CAD build for the part. Positions are in the model's coordinates, mm. A direction names the side the tool comes from. Coordinates: 2 decimals unless noted, no trailing zeros. Order: outer loops, then holes, each group sorted by start corner. A loop starts at its lowest first (then second) coordinate and runs counter-clockwise, first axis right, second up. Notation, with made-up numbers: M 5,66.25 L 55,66.25 A30 cw 55,91.25 Z; hole C 9,44.25 d7. An arc over 180 degrees is marked long. Write item = value, one per line.
from build123d import *

# Parameters (mm, degrees)
SKETCH_W        = 28
SKETCH_H        = 20
SKETCH_R        = 1.75
PAD_DEPTH       = 4
PAD001_DEPTH    = 6
SKETCH002_R     = 3.25
POCKET_DEPTH    = 10
POCKET001_DEPTH = 7
SKETCH004_R     = 8.25
POCKET002_DEPTH = 2


with BuildPart() as part:
    # Sketch → Pad (new body)
    with BuildSketch(Plane.XY):
        Rectangle(SKETCH_W, SKETCH_H)
        with Locations((-11, 0)):
            Circle(SKETCH_R, mode=Mode.SUBTRACT)
        with Locations((11, 0)):
            Circle(SKETCH_R, mode=Mode.SUBTRACT)
    extrude(amount=PAD_DEPTH)

    # Sketch001 (on Face8 of Pad) → Pad001 (join)
    with BuildSketch(Plane.XY.offset(4)):
        with BuildLine():
            ThreePointArc((14, 1.802776), (7.5, 0), (14, -1.802776))
            Line((14, -1.802776), (14, -10))
            Line((14, -10), (-14, -10))
            Line((-14, -10), (-14, -1.802776))
            ThreePointArc((-14, -1.802776), (-7.5, 0), (-14, 1.802776))
            Line((-14, 1.802776), (-14, 10))
            Line((-14, 10), (14, 10))
            Line((14, 10), (14, 1.802776))
        make_face()
    extrude(amount=PAD001_DEPTH)

    # Sketch002 (on Face15 of Pad001) → Pocket (cut)
    with BuildSketch(Plane.XY.offset(10)):
        with Locations((0, 2)):
            Circle(SKETCH002_R)
    extrude(amount=-POCKET_DEPTH, mode=Mode.SUBTRACT)

    # Sketch003 (on Face4 of Pocket) → Pocket001 (cut)
    with BuildSketch(Plane(origin=(0, 0, 0), x_dir=(1, 0, 0), z_dir=(0, 0, -1))):
        Polygon((4.25, -4.453739), (4.25, 0.453739), (0, 2.907477), (-4.25, 0.453739), (-4.25, -4.453739), (0, -6.907477), align=None)
    extrude(amount=-POCKET001_DEPTH, mode=Mode.SUBTRACT)

    # Sketch004 (on Face4 of Pocket001) → Pocket002 (cut)
    with BuildSketch(Plane(origin=(0, 0, 0), x_dir=(1, 0, 0), z_dir=(0, 0, -1))):
        with Locations((0, -2)):
            Circle(SKETCH004_R)
    extrude(amount=-POCKET002_DEPTH, mode=Mode.SUBTRACT)


solid = part.part
(1) Tool access for faces 4 (the face through (0, -2, 10)), 5 (the face through (2, 5, 7)), 6 (the face through (-9, -1, 4)): list every direction of +Z, -Z, +X, -X, +Y, -Y with a clear straight run to the whole face (end or side of a thin tool).
Evaluation:
face_4 = +Z, +X, -X, +Y, -Y
face_5 = -Z
face_6 = +Z
(2) Pull direction X, two halves, no side cores. Call faces 1 (the face through (-2, -2, 2)), 2 (the face through (0, -10, 5)), 3 (the face through (14, 0.1, 3.8)): +X half, -X half, draft (parallel to the pull), parting line (faces both ways), or undercut.
Evaluation:
face_1 = undercut
face_2 = draft
face_3 = +X half
(3) Wall check: line 1 (Y direction, x = 11, z = 3.25); line 2 (X direction, y = -0.75, z = 3.25); line 3 (X direction, y = 2, z = 0.7). Give the ranges that are in metal, low to high. Write a range as from..to.
Evaluation:
line_1 = -10..-1.75, 1.75..10
line_2 = -14..-12.58, -9.42..-3.74, 3.74..9.42, 12.58..14
line_3 = -14..-8.25, 8.25..14
(4) Slice it at A-A, the plane x = -11. Write the cut outline in (y, z).
Evaluation:
outline = M -10,0 L -1.75,0 L -1.75,4 L -3.5,4 L -3.5,10 L -10,10 Z; M 1.75,0 L 10,0 L 10,10 L 3.5,10 L 3.5,4 L 1.75,4 Z
(5) Slice it at C-C, the plane x = 0.75. Write the cut outline in (y, z).
Evaluation:
outline = M -10,0 L -6.22,0 L -6.22,2 L -2.47,2 L -2.47,7 L -1.16,7 L -1.16,10 L -10,10 Z; M 5.16,7 L 6.47,7 L 6.47,2 L 10,2 L 10,10 L 5.16,10 Z
(6) Slice it at B-B, the plane y = 0.75. Write the cut outline in (x, z).
Evaluation:
outline = M -14,0 L -12.58,0 L -12.58,4 L -14,4 Z; M -9.42,0 L -8.15,0 L -8.15,2 L -4.25,2 L -4.25,7 L -3,7 L -3,10 L -7.58,10 L -7.58,4 L -9.42,4 Z; M 3,7 L 4.25,7 L 4.25,2 L 8.15,2 L 8.15,0 L 9.42,0 L 9.42,4 L 7.58,4 L 7.58,10 L 3,10 Z; M 12.58,0 L 14,0 L 14,4 L 12.58,4 Z
(7) Pin check, flat tips, straight feed: pin 1 Ø4.5 at (x, y) = (0.5, 1.5) entering from -Z; pin 2 Ø6 at (x, y) = (2.5, -5) entering from -Z; pin 3 Ø2 at (x, y) = (-12, 1.5) entering from +Z; pin 4 Ø5 at (x, y) = (3.5, 2.5) entering from -Z. Stop position of each tip, or through.
Evaluation:
pin_1 = through
pin_2 = 0
pin_3 = 4
pin_4 = 2
